Check sheet for the modelled part. Datum: model origin and axes. Units: mm. A direction names the side the tool comes from. Give positions to 0.01 mm unless a question says otherwise; leave off trailing zeros. Order: outer loops, then holes, each group sorted by start corner. A loop starts at its lowest first (then second) coordinate and runs counter-clockwise, first axis right, second up.
```python
from build123d import *

# Parameters (mm, degrees)
F0_W     = 40.4834784567
F0_H     = 26.4106485993
F1_DEPTH = 2
F2_W     = 3.0844565481
F2_H     = 3.0844546854
F3_DEPTH = 29.1
F4_R     = 3.0112955683
F5_DEPTH = 9.6
F6_T     = -0.4


with BuildPart() as f1:
    # F0 (on Top) → F1 (new body)
    with BuildSketch(Plane.XY):
        Rectangle(F0_W, F0_H)
    extrude(amount=F1_DEPTH)

    # F2 (on face) → F3 (join)
    with BuildSketch(Plane.XY.offset(2)):
        with Locations((-18.6995109543, 11.6630969569)):
            Rectangle(F2_W, F2_H)
        with Locations((18.6995109543, 11.6630969569)):
            Rectangle(F2_W, F2_H)
        with Locations((18.6995109543, -11.6630969569)):
            Rectangle(F2_W, F2_H)
        with Locations((-18.6995109543, -11.6630969569)):
            Rectangle(F2_W, F2_H)
    extrude(amount=-F3_DEPTH)

    # F4 (on Top) → F5 (join)
    with BuildSketch(Plane.XY):
        with Locations((-15.2294989675, 7.8075276688)):
            Circle(F4_R)
    extrude(amount=F5_DEPTH)

    # F6
    f6_openings = [f1.faces().sort_by_distance(p)[0] for p in [
        (-15.229499, 7.807528, 9.6),
    ]]
    offset(amount=F6_T, openings=f6_openings, kind=Kind.INTERSECTION)


solid = f1.part
```
(1) Tool access check on faces 4 (the face through (19, 10.521, -13)), 5 (the face through (-17.157, -12, -13)), 6 (the face through (-19, 12, -27.1)), 7 (the face through (-19, 10.121, -13)). Record the directions out of +Z, -Z, +X, -X, +Y, -Y that give a thin tool (end or side, any length) a straight path to the whole face; none if there is none.
(2) Sectioned sample at C-C (x = -2.5). Enter the section's corners in (y, z), plus the area to 3 significant figures.
(3) Sectioned sample at D-D (y = 9.5). Enter the section's corners in (x, z), plus the area to 3 significant figures.
(4) Sectioned sample at B-B (y = 2.75). Enter the section's corners in (x, z), plus the area to 3 significant figures.
(5) Thickness scan on L1, parallel to X at y = 10.75, z = -5.5; L2, parallel to Y at x = -18, z = -20; L3, parallel to Z at x = -16.5, y = -7.75. Record the ranges inside material, lowest first.
(6) Go/stop test with flat-tipped pins: P1, Ø1, axis at x = 2, y = 4, coming from the -Z side; P2, Ø6, axis at x = 15.5, z = -4.5, coming from the +Y side; P3, Ø1.1, axis at x = 19, y = -12, coming from the +Z side; P4, Ø3, axis at x = -15.23, y = 7.81, coming from the +Z side. Record where each tip stops, or that it passes through.
(7) Sectioned sample at A-A (z = -20.5). Count the separate pieces of the cut face and the enclosed holes in it, plus the area to 3 significant figures.
(8) Release check for a two-part mould opening along X. For faces 1 (the face through (19, 10.121, -13)), 2 (the face through (-14.025, 5.491, 5.544)), 3 (the face through (-15.622, 10.793, 5.747)) record: released by +X, released by -X, zero draft, split by the parting line, or undercut.
Values follow:
1. face 4: none
1. face 5: -Z, +Y, -Y
1. face 6: -Z, +X, -X, +Y, -Y
1. face 7: -Z, +X, -X
2. outline: (-13.21, 0) - (13.21, 0) - (13.21, 2) - (-13.21, 2) - close; hole (-12.81, 0.4) - (12.81, 0.4) - (12.81, 1.6) - (-12.81, 1.6) - close
2. area: 22.1 mm2
3. outline: (-20.24, 0) - (20.24, 0) - (20.24, 2) - (-12.74, 2) - (-12.74, 9.6) - (-13.24, 9.6) - (-13.24, 1.6) - (19.84, 1.6) - (19.84, 0.4) - (-19.84, 0.4) - (-19.84, 1.6) - (-17.22, 1.6) - (-17.22, 9.6) - (-17.72, 9.6) - (-17.72, 2) - (-20.24, 2) - close
3. area: 39.4 mm2
4. outline: (-20.24, 0) - (20.24, 0) - (20.24, 2) - (-20.24, 2) - close; hole (-19.84, 0.4) - (19.84, 0.4) - (19.84, 1.6) - (-19.84, 1.6) - close
4. area: 33.3 mm2
5. L1: x = -20.24 to -19.84, -17.56 to -17.16, 17.16 to 17.56, 19.84 to 20.24
5. L2: y = -13.21 to -12.81, -10.52 to -10.12, 10.12 to 10.52, 12.81 to 13.21
5. L3: z = 0 to 0.4, 1.6 to 2
6. P1: stops at z = 0
6. P2: stops at y = 13.21
6. P3: stops at z = 2
6. P4: stops at z = 0.4
7. separate pieces: 4
7. enclosed holes: 4
7. area: 17.2 mm2
8. face 1: zero draft
8. face 2: undercut
8. face 3: split by the parting line
